from build123d import *

# Parameters (mm, degrees)
CROQUIS2_W              = 14
CROQUIS2_H              = 31
CROQUIS2_R              = 1.55
SALIENTE_EXTRUIR1_DEPTH = 50
CROQUIS3_W              = 26
CROQUIS3_H              = 45
CORTAR_EXTRUIR1_DEPTH   = 14
CORTAR_EXTRUIR2_DEPTH   = 5
CORTAR_EXTRUIR3_DEPTH   = 1.5
SALIENTE_EXTRUIR3_DEPTH = 14
CROQUIS7_OUTSIDE_W      = 28.094
CROQUIS7_OUTSIDE_H      = 45.094
CORTAR_EXTRUIR5_DEPTH   = 45
REDONDEO1_R             = 2
CROQUIS8_W              = 12.5
CROQUIS8_H              = 0.5
CORTAR_EXTRUIR6_DEPTH   = 50


with BuildPart() as part:
    # Croquis2 → Saliente-Extruir1 (new body)
    with BuildSketch(Plane(origin=(0, 0, 0), x_dir=(1, 0, 0), z_dir=(0, 1, 0))):
        with Locations((7, 15.5)):
            Rectangle(CROQUIS2_W, CROQUIS2_H)
        with Locations((7, 22)):
            Circle(CROQUIS2_R, mode=Mode.SUBTRACT)
        with Locations((7, 4)):
            Circle(CROQUIS2_R, mode=Mode.SUBTRACT)
    extrude(amount=SALIENTE_EXTRUIR1_DEPTH)

    # Croquis3 → Cortar-Extruir1 (cut)
    with BuildSketch(Plane.ZY):
        with Locations((-13, 27.5)):
            Rectangle(CROQUIS3_W, CROQUIS3_H)
    extrude(amount=-CORTAR_EXTRUIR1_DEPTH, mode=Mode.SUBTRACT)

    # Croquis4 → Cortar-Extruir2 (cut)
    with BuildSketch(Plane(origin=(0, 0, -31), x_dir=(-1, 0, 0), z_dir=(0, 0, -1))):
        with BuildLine():
            Line((-8.55, 8), (-8.55, 18))
            ThreePointArc((-8.55, 18), (-7, 19.55), (-5.45, 18))
            Line((-5.45, 18), (-5.45, 8))
            ThreePointArc((-5.45, 8), (-7, 6.45), (-8.55, 8))
        make_face()
        with BuildLine():
            Line((-8.55, 32), (-8.55, 42))
            ThreePointArc((-8.55, 42), (-7, 43.55), (-5.45, 42))
            Line((-5.45, 42), (-5.45, 32))
            ThreePointArc((-5.45, 32), (-7, 30.45), (-8.55, 32))
        make_face()
    extrude(amount=-CORTAR_EXTRUIR2_DEPTH, mode=Mode.SUBTRACT)

    # Croquis5 → Cortar-Extruir3 (cut)
    with BuildSketch(Plane(origin=(0, 5, 0), x_dir=(1, 0, 0), z_dir=(0, 1, 0))):
        Polygon((10.348631561, 4), (8.674315781, 6.9), (5.325684219, 6.9), (3.651368439, 4), (5.325684219, 1.1), (8.674315781, 1.1), align=None)
        Polygon((8.674315781, 19.1), (10.348631561, 22), (8.674315781, 24.9), (5.325684219, 24.9), (3.651368439, 22), (5.325684219, 19.1), align=None)
    extrude(amount=-CORTAR_EXTRUIR3_DEPTH, mode=Mode.SUBTRACT)

    # Croquis6 → Saliente-Extruir3 (add)
    with BuildSketch(Plane.ZY):
        with BuildLine():
            Line((-26, 5), (-26, 35))
            ThreePointArc((-26, 35), (-20.21590319, 16.698867767), (-5, 5))
            Line((-5, 5), (-26, 5))
        make_face()
    extrude(amount=-SALIENTE_EXTRUIR3_DEPTH)

    # Croquis7 outside → Cortar-Extruir5 (cut)
    with BuildSketch(Plane(origin=(0, 50, 0), x_dir=(1, 0, 0), z_dir=(0, 1, 0))):
        with Locations((7, 15.5)):
            Rectangle(CROQUIS7_OUTSIDE_W, CROQUIS7_OUTSIDE_H)
        Polygon((0, 26), (0, 0), (3, 0), (3, 26), (11, 26), (11, 0), (14, 0), (14, 26), (14, 31), (0, 31), align=None, mode=Mode.SUBTRACT)
    extrude(amount=-CORTAR_EXTRUIR5_DEPTH, mode=Mode.SUBTRACT)

    # Redondeo1
    redondeo1_edges = [part.edges().sort_by_distance(p)[0] for p in [
        (14, 2.5, 0),
        (0, 2.5, 0),
    ]]
    fillet(redondeo1_edges, radius=REDONDEO1_R)

    # Croquis8 → Cortar-Extruir6 (cut)
    with BuildSketch(Plane(origin=(0, 50, 0), x_dir=(1, 0, 0), z_dir=(0, 1, 0))):
        with Locations((7, 30.75)):
            Rectangle(CROQUIS8_W, CROQUIS8_H)
    extrude(amount=-CORTAR_EXTRUIR6_DEPTH, mode=Mode.SUBTRACT)


solid = part.part
Source: CAD feature listing. Evaluate the final solid. Frame: model axes, mm. A direction names the side the tool comes from. Round coordinates to 2 decimals unless told otherwise and drop trailing zeros. Loops run counter-clockwise (first coordinate to the right, second up) from the corner with the lowest first, then second, coordinate; pieces in that order, holes last. Notation, with made-up numbers: (30, 33.5) -> (68, 33.5) arc R28 cw to (68, 70.5) -> close; hole circle Ø11 at (-27.75, 47). An arc over 180 degrees is marked (long way). Answer as a JSON object with one key per item and string values. Group by question number.
Q1. Section query A-A (y = 39.5). Output: boundary loops of the cut face in (x, z), plus the area to 3 significant figures.
Q2. Section query B-B (z = -27). Output: boundary loops of the cut face in (x, y).
Q3. Section query D-D (y = 44.5). Output: boundary loops of the cut face in (x, z).
Q4. Ray query, line 1 (Z direction, x = 7, y = 1.55); line 2 (X direction, y = 1, z = -22); line 3 (X direction, y = 7, z = -25). Return the intervals inside material, ascending. Write a range as from..to.
Q5. Access query for faces 4 (the cylindrical face through (7.03, 19.55, -28.28)), 5 (the flat face through (8.4, 3.5, -5.3)), 6 (the flat face through (7, 25, -30.5)), 7 (the flat face through (5, 33, -26)). Directions: +Z, -Z, +X, -X, +Y, -Y. A direction counts if a zero-diameter tool reaches every point of the face in a straight line with its end or side. Return the directions, or none.
Q6. Mould query, pull axis Y, two halves, no side actions, for faces 1 (the flat face through (7, 4, -24.9)), 2 (the flat face through (7, 0, -16)), 3 (the flat face through (8.55, 37, -28)). Classes: pulls with the +Y half, pulls with the -Y half, needs draft (parallel to the pull), parting line crosses it, or undercut.
Q7. Contact query for flat-ended pins moving along their axis: P1, Ø1, axis at x = 4, y = 41, coming from the +Z side; P2, Ø6.5, axis at y = 25, z = -19.5, coming from the +X side; P3, Ø1.2, axis at x = 7.5, y = 4.5, coming from the -Z side; P4, Ø6, axis at x = 12.5, y = 31.5, coming from the +Z side. Output: stop coordinate, or through.
Q8. Section query C-C (x = 7). State how many separate pieces and enclosed holes the cut face has, plus the area to 3 significant figures.
Completed:
{
 "1": {"outline": "(0, -31) -> (0.75, -31) -> (0.75, -30.5) -> (5.45, -30.5) -> (5.45, -26) -> (0, -26) -> close; (8.55, -30.5) -> (13.25, -30.5) -> (13.25, -31) -> (14, -31) -> (14, -26) -> (8.55, -26) -> close", "area": "49.8 mm²"},
 "2": {"outline": "(0, 0) -> (14, 0) -> (14, 50) -> (0, 50) -> close; hole (5.45, 8) arc R1.55 ccw to (8.55, 8) -> (8.55, 18) arc R1.55 ccw to (5.45, 18) -> close; hole (5.45, 32) arc R1.55 ccw to (8.55, 32) -> (8.55, 42) arc R1.55 ccw to (5.45, 42) -> close"},
 "3": {"outline": "(0, -31) -> (0.75, -31) -> (0.75, -30.5) -> (13.25, -30.5) -> (13.25, -31) -> (14, -31) -> (14, -26) -> (0, -26) -> close"},
 "4": {"line 1": "-30.5..-23.55, -20.45..-5.55, -2.45..0", "line 2": "0..5.45, 8.55..14", "line 3": "0..3, 11..14"},
 "5": {"face 4": "+Z, -Z", "face 5": "+Y", "face 6": "-Z, +Y, -Y", "face 7": "+Z, +Y"},
 "6": {"face 1": "needs draft", "face 2": "pulls with the -Y half", "face 3": "undercut"},
 "7": {"P1": "z = -26", "P2": "through", "P3": "z = -30.5", "P4": "z = -25.32"},
 "8": {"separate pieces": "5", "enclosed holes": "0", "area": "198 mm²"}
}
